Part print with two shaded views. Sizes in mm from the minimum x, y, z corner. Give positions to 0.01 mm unless a question says otherwise; leave off trailing zeros. Write each loop counter-clockwise with the first axis right and the second up, starting at its lowest first coordinate (ties: lowest second). Pieces come first, ordered by that corner, then holes. Notation, with made-up numbers: (48.5, 52.5) -> (84.5, 52.5) arc R34 cw to (84.5, 84.5) -> close; hole circle Ø10 at (-32.5, 9.5). An arc over 180 degrees is marked (long way). Answer in a Markdown table with one row per item. Add a question column.
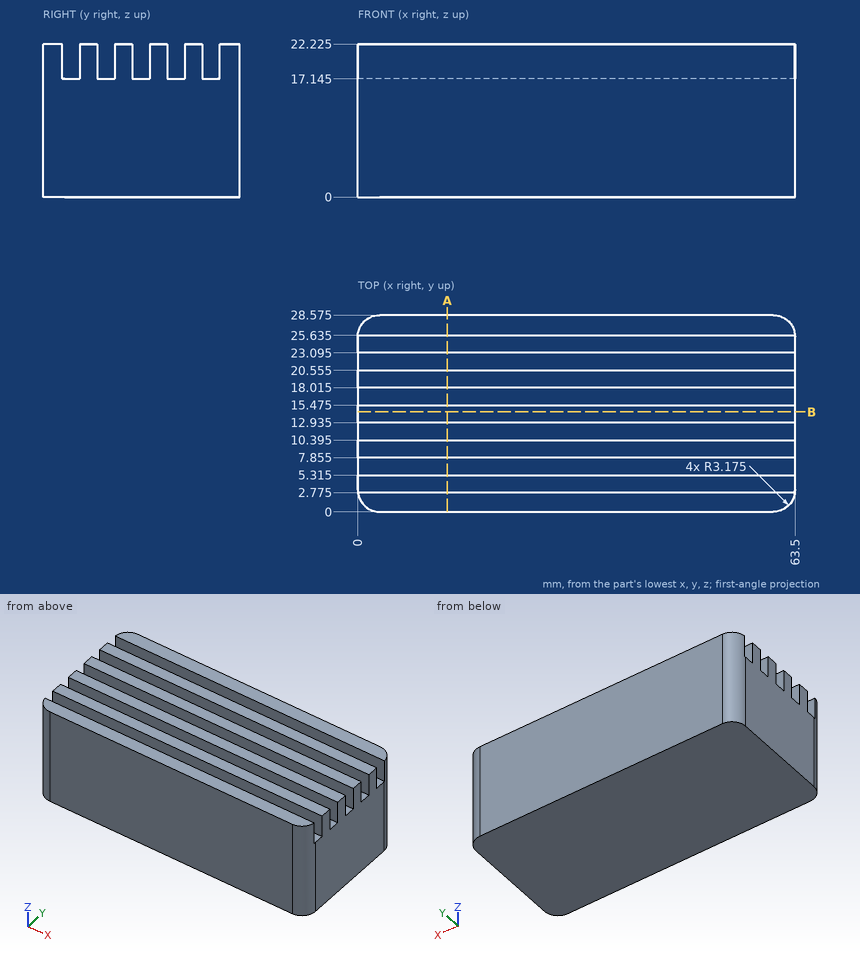
Item 1: Slice it at B-B, the plane y = 14.5. List the corners of the cut face in (x, z) (3 decimals).
Item 2: Drop a flat-ended pin along its axis: pin 1 Ø0.8 at (x, y) = (46, 4) entering from +Z (3 decimals). Give the stop position or say it passes through.
Item 3: Slice it at A-A, the plane x = 13. List the corners of the cut face in (y, z) (3 decimals).
Item 4: Probe L1, parallel to Y at x = 50, z = 20 (3 decimals); L2, parallel to Z at x = 12, y = 8 (3 decimals); L3, parallel to X at y = 26.25, z = 10. List the from-to ranges inside material, lowest first. Write a range as from..to.
Answer key:
| question | item | result |
|---|---|---|
| 1 | outline | (0, 0) -> (63.5, 0) -> (63.5, 17.145) -> (0, 17.145) -> close |
| 2 | pin 1 | stops at z = 17.145 |
| 3 | outline | (0, 0) -> (28.575, 0) -> (28.575, 22.225) -> (25.635, 22.225) -> (25.635, 17.145) -> (23.095, 17.145) -> (23.095, 22.225) -> (20.555, 22.225) -> (20.555, 17.145) -> (18.015, 17.145) -> (18.015, 22.225) -> (15.475, 22.225) -> (15.475, 17.145) -> (12.935, 17.145) -> (12.935, 22.225) -> (10.395, 22.225) -> (10.395, 17.145) -> (7.855, 17.145) -> (7.855, 22.225) -> (5.315, 22.225) -> (5.315, 17.145) -> (2.775, 17.145) -> (2.775, 22.225) -> (0, 22.225) -> close |
| 4 | L1 | y = 0..2.775, 5.315..7.855, 10.395..12.935, 15.475..18.015, 20.555..23.095, 25.635..28.575 |
| 4 | L2 | z = 0..17.145 |
| 4 | L3 | x = 0.12..63.38 |
